The listing builds one solid part. Answer for the finished solid, in the listing's coordinates (mm). A direction names the side the tool comes from. Coordinates: 2 decimals unless noted, no trailing zeros. Order: outer loops, then holes, each group sorted by start corner. A loop starts at its lowest first (then second) coordinate and runs counter-clockwise, first axis right, second up. Notation, with made-up numbers: (87, 9.5) -> (95, 9.5) arc R20 ccw to (95, 14.5) -> close; hole circle Ø8 at (-9.75, 64.5). An arc over 180 degrees is marked (long way). Return JSON: item names as keys, results as strings.
```python
from build123d import *

# Parameters (mm, degrees)
F1_DEPTH = 3
F2_R     = 1.5
F3_DEPTH = 25
F6_DEPTH = 2
F9_DEPTH = 2


with BuildPart() as f1:
    # F0 (on Front) → F1 (new body)
    with BuildSketch(Plane.XZ):
        Polygon((-1.443376, -2.5), (1.443376, -2.5), (2.886751, 0), (1.443376, 2.5), (-1.443376, 2.5), (-2.886751, 0), align=None)
    extrude(amount=F1_DEPTH)

    # F2 (on face) → F3 (join)
    with BuildSketch(Plane(origin=(0, 0, 0), x_dir=(-1, 0, 0), z_dir=(0, 1, 0))):
        Circle(F2_R)
    extrude(amount=F3_DEPTH)

    # F5 (on offset) → F6 (join)
    with BuildSketch(Plane.XZ.offset(-15)):
        Polygon((1.437224, 2.489345), (-1.437224, 2.489345), (-2.874448, 0), (-1.437224, -2.489345), (1.437224, -2.489345), (2.874448, 0), align=None)
    extrude(amount=-F6_DEPTH)

    # F8 (on offset) → F9 (join)
    with BuildSketch(Plane.XZ.offset(-17)):
        Polygon((2.5, -1.443376), (2.5, 1.443376), (0, 2.886751), (-2.5, 1.443376), (-2.5, -1.443376), (0, -2.886751), align=None)
    extrude(amount=-F9_DEPTH)


solid = f1.part
```
Item 1: The part is cut by section B-B on y = -1. Determine the outline of the cut face in (x, z).
Answer list:
{"outline": "(-2.89, 0) -> (-1.44, -2.5) -> (1.44, -2.5) -> (2.89, 0) -> (1.44, 2.5) -> (-1.44, 2.5) -> close"}
Item 2: Which of the six approach directions +Z, -Z, +X, -X, +Y, -Y give full straight-line access (tool end or side, diameter ignored) to faces 4 (the flat face through (1.267, 17.986, 2.155)), 5 (the cylindrical face through (1.5, 7.4, 0.07)), 6 (the flat face through (-1.233, 17.986, 2.175))?
Answer list:
{"face 4": "+Z, +X, +Y", "face 5": "none", "face 6": "+Z, -X, +Y"}
Item 3: Flat-ended cylindrical pins translate along their axes: pin 1 (2.5 mm diameter, centred on x = -0.5, y = -2, fed in from -Z); pin 2 (1.4 mm diameter, centred on x = 0.5, y = -1.5, fed in from +Z). Find the tip coordinate at first contact, or state that the pin passes through.
Answer list:
{"pin 1": "z = -2.5", "pin 2": "z = 2.5"}
Item 4: The part is cut by section C-C on x = 1.05. Determine the outline of the cut face in (y, z), plus the area to 3 significant figures.
Answer list:
{"outline": "(-3, -2.5) -> (0, -2.5) -> (0, -1.07) -> (15, -1.07) -> (15, -2.49) -> (17, -2.49) -> (17, -2.28) -> (19, -2.28) -> (19, -1.07) -> (25, -1.07) -> (25, 1.07) -> (19, 1.07) -> (19, 2.28) -> (17, 2.28) -> (17, 2.49) -> (15, 2.49) -> (15, 1.07) -> (0, 1.07) -> (0, 2.5) -> (-3, 2.5) -> close", "area": "79.1 mm2"}
Item 5: The part is cut by section D-D on y = 14. Determine the outline of the cut face in (x, z), plus the area to 3 significant figures.
Answer list:
{"outline": "circle Ø3 at (0, 0)", "area": "7.07 mm2"}
Item 6: Find the intervals of material crossed by probe 1 along Y at (x, z) = (1.2, 1.55); probe 2 along X at (y, z) = (20.25, -0.4); probe 3 along X at (y, z) = (8.75, -0.1), in increasing order.
Answer list:
{"probe 1": "-3 to 0, 15 to 19", "probe 2": "-1.45 to 1.45", "probe 3": "-1.5 to 1.5"}
Item 7: The part is cut by section A-A on z = 2.25. Determine the outline of the cut face in (x, y), plus the area to 3 significant figures.
Answer list:
{"outline": "(-1.59, -3) -> (1.59, -3) -> (1.59, 0) -> (-1.59, 0) -> close; (-1.58, 15) -> (1.58, 15) -> (1.58, 17) -> (1.1, 17) -> (1.1, 19) -> (-1.1, 19) -> (-1.1, 17) -> (-1.58, 17) -> close", "area": "20.2 mm2"}
Item 8: Determine the mould class of faces 1 (the flat face through (1.24, 15, 1.14)), 2 (the flat face through (0, 25, 0)), 3 (the flat face through (0, -1, 2.5)) for opening direction Y: pulls with the +Y half, pulls with the -Y half, needs draft (parallel to the pull), parting line crosses it, or undercut.
Answer list:
{"face 1": "undercut", "face 2": "pulls with the +Y half", "face 3": "needs draft"}
